For this review, take the finished solid that the model builds, in its own axes (mm). Face numbers are marked on the shaded views. A direction names the side the tool comes from. Coordinates: 2 decimals unless noted, no trailing zeros. Loops run counter-clockwise (first coordinate to the right, second up) from the corner with the lowest first, then second, coordinate; pieces in that order, holes last. Notation, with made-up numbers: (-7, -15.5) - (36, -15.5) arc R25 ccw to (36, 4.5) - close; hole circle Ø2 at (12.5, 65). An arc over 180 degrees is marked (long way). One line per item, written item: value. Start each with the question number.
1. To check wall thickness, follow line 1 (Y direction, x = 5, z = 0); line 2 (X direction, y = 3, z = -2.5) (3 decimals); line 3 (Y direction, x = -1.5, z = 0.25). State the ranges of each line that lie inside material, in increasing order. Write a range as from..to.
2. For the marked faces 1, 2, 3, 4 and 5, list the 3-axis set-ups (+Z, -Z, +X, -X, +Y, -Y) from which the entire face can be reached by the end or side of a thin tool; tool diameter is ignored.
3. Take a section at C-C, the plane y = 4.75. State the section outline as (x, z) points (3 decimals).
4. Insertion check: pin 1 (3 mm diameter, centred on x = 2, y = 3.5, fed in from -Z); pin 2 (1.4 mm diameter, centred on y = 4.5, z = 0.5, fed in from -X) (3 decimals). Each pin has a flat end and moves straight along its axis. Give the tip position at first contact, or say it passes through.
5. Take a section at D-D, the plane x = -4. State the section outline as (y, z) points (3 decimals), and give its area (3 significant figures).
6. Take a section at A-A, the plane z = 0.5. State the section outline as (x, y) points (3 decimals), and give its area (3 significant figures).
7. Take a section at B-B, the plane x = -0.25. State the section outline as (y, z) points (3 decimals), and give its area (3 significant figures).
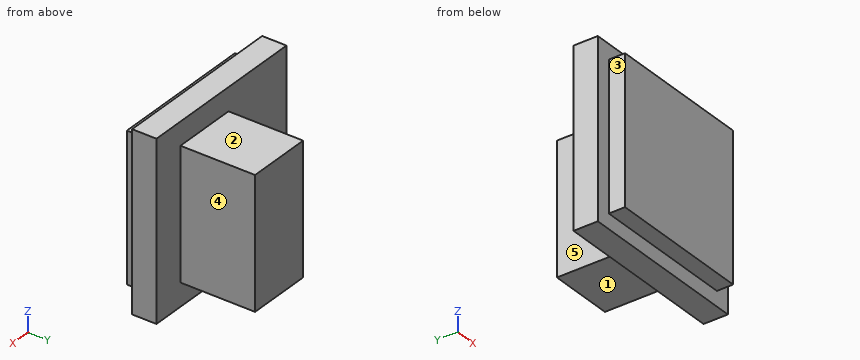
```python
from build123d import *

# Parameters (mm, degrees)
SKETCH1_W      = 10.83
SKETCH1_H      = 10.83
EXTRUDE1_DEPTH = 1.5
SKETCH2_W      = 9
SKETCH2_H      = 9
EXTRUDE2_DEPTH = 1
SKETCH3_W      = 4
SKETCH3_H      = 8
EXTRUDE3_DEPTH = 4.6


with BuildPart() as part:
    # Sketch1 → Extrude1 (new body)
    with BuildSketch(Plane(origin=(0, 0, 0), x_dir=(1, 0, 0), z_dir=(0, 1, 0))):
        Rectangle(SKETCH1_W, SKETCH1_H)
    extrude(amount=EXTRUDE1_DEPTH)

    # Sketch2 → Extrude2 (add)
    with BuildSketch(Plane.XZ):
        Rectangle(SKETCH2_W, SKETCH2_H)
    extrude(amount=EXTRUDE2_DEPTH)

    # Sketch3 → Extrude3 (add)
    with BuildSketch(Plane(origin=(0, 1.5, 0), x_dir=(1, 0, 0), z_dir=(0, 1, 0))):
        with Locations((1.415, 0)):
            Rectangle(SKETCH3_W, SKETCH3_H)
    extrude(amount=EXTRUDE3_DEPTH)


solid = part.part
```
Solutions:
1. line 1: 0..1.5
1. line 2: -0.585..3.415
1. line 3: -1..1.5
2. face 1: -Z, +X, -X, +Y
2. face 2: +Z, +X, -X, +Y
2. face 3: +Z, -Z, -X, -Y
2. face 4: +Z, -Z, +X, +Y
2. face 5: +Z, -Z, -X, +Y
3. outline: (-0.585, -4) - (3.415, -4) - (3.415, 4) - (-0.585, 4) - close
4. pin 1: z = -4
4. pin 2: x = -0.585
5. outline: (-1, -4.5) - (0, -4.5) - (0, -5.415) - (1.5, -5.415) - (1.5, 5.415) - (0, 5.415) - (0, 4.5) - (-1, 4.5) - close
5. area: 25.2 mm2
6. outline: (-5.415, 0) - (-4.5, 0) - (-4.5, -1) - (4.5, -1) - (4.5, 0) - (5.415, 0) - (5.415, 1.5) - (3.415, 1.5) - (3.415, 6.1) - (-0.585, 6.1) - (-0.585, 1.5) - (-5.415, 1.5) - close
6. area: 43.6 mm2
7. outline: (-1, -4.5) - (0, -4.5) - (0, -5.415) - (1.5, -5.415) - (1.5, -4) - (6.1, -4) - (6.1, 4) - (1.5, 4) - (1.5, 5.415) - (0, 5.415) - (0, 4.5) - (-1, 4.5) - close
7. area: 62.0 mm2
